Part print with two shaded views. Sizes in mm from the minimum x, y, z corner. Round coordinates to 2 decimals unless told otherwise and drop trailing zeros. Write each loop counter-clockwise with the first axis right and the second up, starting at its lowest first coordinate (ties: lowest second). Pieces come first, ordered by that corner, then holes. Notation, with made-up numbers: M 84.25,36.5 L 124.25,36.5 A33 ccw 124.25,71.5 Z; hole C 51,-18 d6. An arc over 180 degrees is marked long. One line per question, with ' | ' between items. Start each with the question number.
1) Saw through at B-B (x = 5). List the corners of the cut face in (y, z).
2) Saw through at C-C (z = 2.25). Give the number of separate pieces and of enclosed holes in the cut face, plus the area to 3 significant figures.
3) Saw through at D-D (x = 11). List the corners of the cut face in (y, z), plus the area to 3 significant figures.
4) Saw through at A-A (y = 3). List the corners of the cut face in (x, z).
5) Drop a flat-ended pin along its axis: pin 1 Ø0.9 at (x, z) = (22, 1) entering from -Y. Give the stop position or say it passes through.
6) Wall check: probe 1 along Y at (x, z) = (55, 2); probe 2 along X at (y, z) = (15.25, 2.35); probe 3 along Y at (x, z) = (22, 1.8). Give the ranges that are in metal, low to high. Write a range as [from, to].
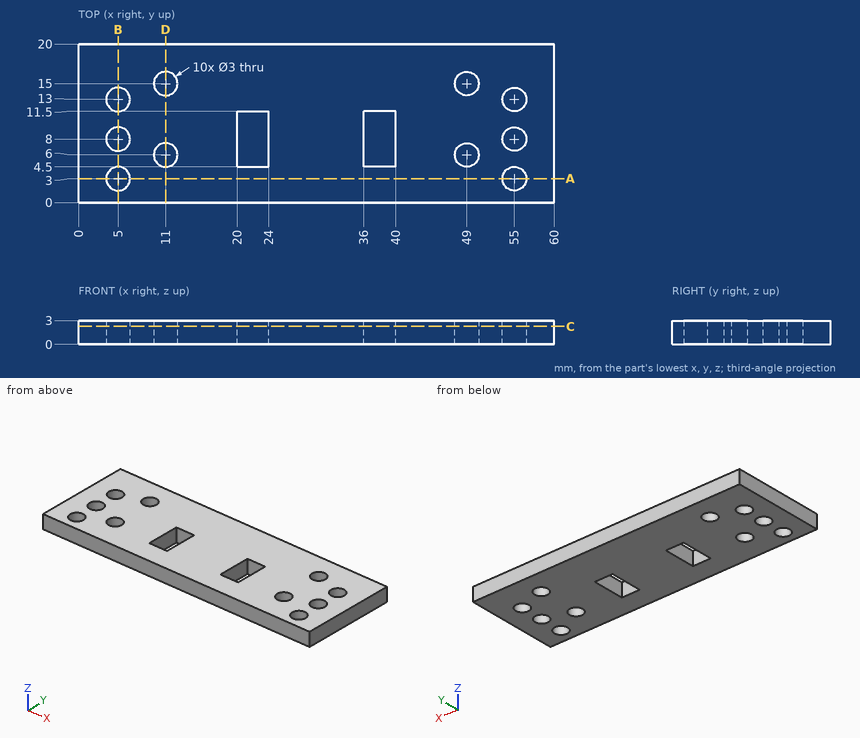
Answer key:
1) outline: M 0,0 L 1.5,0 L 1.5,3 L 0,3 Z; M 4.5,0 L 6.5,0 L 6.5,3 L 4.5,3 Z; M 9.5,0 L 11.5,0 L 11.5,3 L 9.5,3 Z; M 14.5,0 L 20,0 L 20,3 L 14.5,3 Z
2) separate pieces: 1 | enclosed holes: 12 | area: 1,070 mm2
3) outline: M 0,0 L 4.5,0 L 4.5,3 L 0,3 Z; M 7.5,0 L 13.5,0 L 13.5,3 L 7.5,3 Z; M 16.5,0 L 20,0 L 20,3 L 16.5,3 Z | area: 42.0 mm2
4) outline: M 0,0 L 3.5,0 L 3.5,3 L 0,3 Z; M 6.5,0 L 53.5,0 L 53.5,3 L 6.5,3 Z; M 56.5,0 L 60,0 L 60,3 L 56.5,3 Z
5) pin 1: stops at y = 0
6) probe 1: y = [0, 1.5], [4.5, 6.5], [9.5, 11.5], [14.5, 20] | probe 2: x = [0, 9.52], [12.48, 47.52], [50.48, 60] | probe 3: y = [0, 4.5], [11.5, 20]
